Verification items for this drawing (mm, ordinates from the low corner). A direction names the side the tool comes from. Give positions to 0.01 mm unless a question says otherwise; leave off trailing zeros. Write each loop counter-clockwise with the first axis right and the second up, starting at its lowest first coordinate (ties: lowest second). Pieces come first, ordered by that corner, then holes. Notation, with made-up numbers: (10.25, 69.5) -> (32.25, 69.5) arc R22 ccw to (32.25, 82.5) -> close; hole circle Ø5 at (-8.75, 27.5). An arc over 180 degrees is marked (long way). One line per item, written item: value.
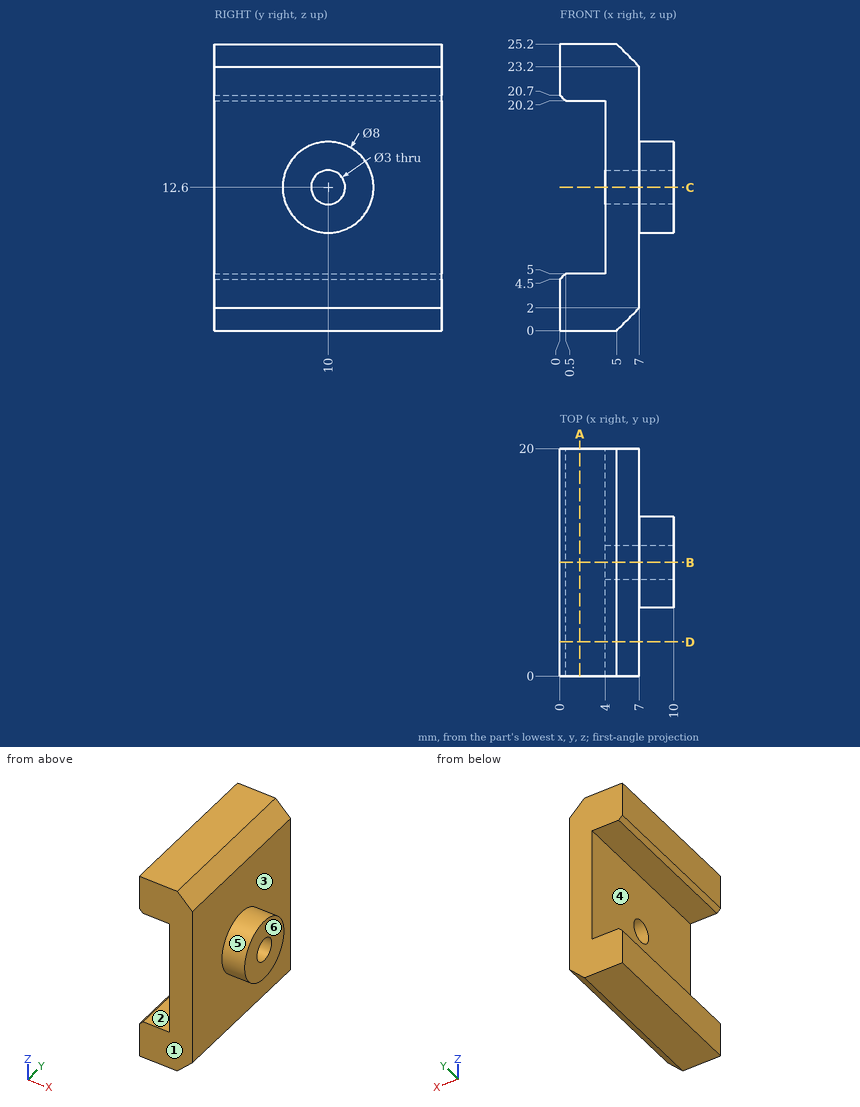
1) Scan lines: probe 1 along Z at (x, y) = (3.25, 2.75); probe 2 along Y at (x, z) = (6.7, 12.6); probe 3 along Y at (x, z) = (8.5, 12.6). Record each from-to range of solid material in increasing order.
Verdict:
probe 1: 0 to 5, 20.2 to 25.2
probe 2: 0 to 8.5, 11.5 to 20
probe 3: 6 to 8.5, 11.5 to 14
2) Sectioned sample at D-D on y = 3. Record the cut outline in (x, z), plus the area to 3 significant figures.
Verdict:
outline: (0, 0) -> (5, 0) -> (7, 2) -> (7, 23.2) -> (5, 25.2) -> (0, 25.2) -> (0, 20.7) -> (0.5, 20.2) -> (4, 20.2) -> (4, 5) -> (0.5, 5) -> (0, 4.5) -> close
area: 111 mm^2
3) Mould release check, pull along Z, two halves, no side actions. Record for the marked faces 4, 5 and 6: released by +Z, released by -Z, zero draft, split by the parting line, or undercut.
Verdict:
face 4: undercut
face 5: split by the parting line
face 6: zero draft
4) Sectioned sample at C-C on z = 12.6. Record the cut outline in (x, y), plus the area to 3 significant figures.
Verdict:
outline: (4, 0) -> (7, 0) -> (7, 6) -> (10, 6) -> (10, 8.5) -> (4, 8.5) -> close; (4, 11.5) -> (10, 11.5) -> (10, 14) -> (7, 14) -> (7, 20) -> (4, 20) -> close
area: 66.0 mm^2
5) Depth check by flat-ended pin: pin 1 Ø1.5 at (x, y) = (7, 3) entering from -Z; pin 2 Ø1 at (y, z) = (8.5, 9.5) entering from -X. Enter the tip coordinate at first touch or a pass-through.
Verdict:
pin 1: z = 1.25
pin 2: x = 4
6) Sectioned sample at A-A on x = 1.75. Record the cut outline in (y, z).
Verdict:
outline: (0, 0) -> (20, 0) -> (20, 5) -> (0, 5) -> close; (0, 20.2) -> (20, 20.2) -> (20, 25.2) -> (0, 25.2) -> close
7) Tool access check on the marked faces 1, 2 and 3. Record the directions out of +Z, -Z, +X, -X, +Y, -Y that give a thin tool (end or side, any length) a straight path to the whole face; none if there is none.
Verdict:
face 1: +Z, -Z, +X, -X, -Y
face 2: -X, +Y, -Y
face 3: +X
8) Sectioned sample at B-B on y = 10. Record the cut outline in (x, z), plus the area to 3 significant figures.
Verdict:
outline: (0, 0) -> (5, 0) -> (7, 2) -> (7, 8.6) -> (10, 8.6) -> (10, 11.1) -> (4, 11.1) -> (4, 5) -> (0.5, 5) -> (0, 4.5) -> close; (0, 20.7) -> (0.5, 20.2) -> (4, 20.2) -> (4, 14.1) -> (10, 14.1) -> (10, 16.6) -> (7, 16.6) -> (7, 23.2) -> (5, 25.2) -> (0, 25.2) -> close
area: 117 mm^2
